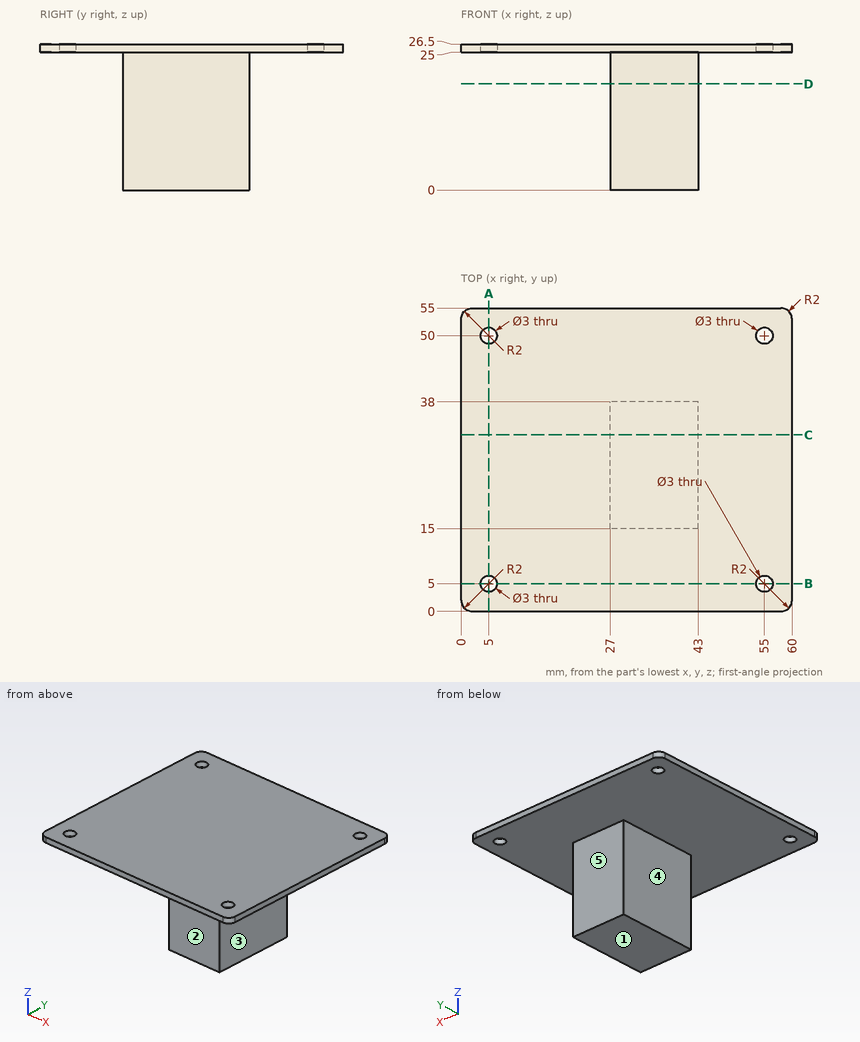
Answer from the drawing. Dimensions are ordinates in mm from the lowest x, y and z of the part. A direction names the side the tool comes from. Coordinates: 2 decimals unless noted, no trailing zeros. Write each loop counter-clockwise with the first axis right and the second up, starting at its lowest first coordinate (ties: lowest second). Pieces come first, ordered by that corner, then holes. Notation, with made-up numbers: (47.5, -5.75) - (90.5, -5.75) arc R15 ccw to (90.5, 16.25) - close; hole circle Ø6 at (77.25, 87). An arc over 180 degrees is marked (long way). Return JSON: item names as keys, results as strings.
1. The part is cut by section D-D on z = 19.25. Determine the outline of the cut face in (x, y).
Final values:
{"outline": "(27, 15) - (43, 15) - (43, 38) - (27, 38) - close"}
2. The part is cut by section B-B on y = 5. Determine the outline of the cut face in (x, z).
Final values:
{"outline": "(0, 25) - (3.5, 25) - (3.5, 26.5) - (0, 26.5) - close; (6.5, 25) - (53.5, 25) - (53.5, 26.5) - (6.5, 26.5) - close; (56.5, 25) - (60, 25) - (60, 26.5) - (56.5, 26.5) - close"}
3. The part is cut by section A-A on x = 5. Determine the outline of the cut face in (y, z), then the cut area to 3 significant figures.
Final values:
{"outline": "(0, 25) - (3.5, 25) - (3.5, 26.5) - (0, 26.5) - close; (6.5, 25) - (48.5, 25) - (48.5, 26.5) - (6.5, 26.5) - close; (51.5, 25) - (55, 25) - (55, 26.5) - (51.5, 26.5) - close", "area": "73.5 mm^2"}
4. Which of the six approach directions +Z, -Z, +X, -X, +Y, -Y give full straight-line access (tool end or side, diameter ignored) to the marked faces 1, 2, 3, 4 and 5?
Final values:
{"face 1": "-Z, +X, -X, +Y, -Y", "face 2": "-Z, +X, -X, -Y", "face 3": "-Z, +X, +Y, -Y", "face 4": "-Z, -X, +Y, -Y", "face 5": "-Z, +X, -X, +Y"}
5. Each of these flat-tipped pins is pushed along its axis until it touches: pin 1 Ø1.5 at (x, y) = (25.5, 25.5) entering from -Z; pin 2 Ø12 at (x, z) = (25.5, 12) entering from -Y; pin 3 Ø1 at (x, z) = (6.5, 23) entering from +Y; pin 4 Ø6 at (y, z) = (22.5, 6) entering from -X. Where does it stop, or does it pass through?
Final values:
{"pin 1": "z = 25", "pin 2": "y = 15", "pin 3": "through", "pin 4": "x = 27"}
6. The part is cut by section C-C on y = 32. Determine the outline of the cut face in (x, z), then the cut area to 3 significant figures.
Final values:
{"outline": "(0, 25) - (27, 25) - (27, 0) - (43, 0) - (43, 25) - (60, 25) - (60, 26.5) - (0, 26.5) - close", "area": "490 mm^2"}
7. Consider line 1 along Y through (x, z) = (55, 25.45); line 2 along Z through (x, y) = (49, 18.5); line 3 along X through (y, z) = (15.5, 3.5). Determine where each line is inside the solid, lowest interval first.
Final values:
{"line 1": "0 to 3.5, 6.5 to 48.5, 51.5 to 55", "line 2": "25 to 26.5", "line 3": "27 to 43"}
